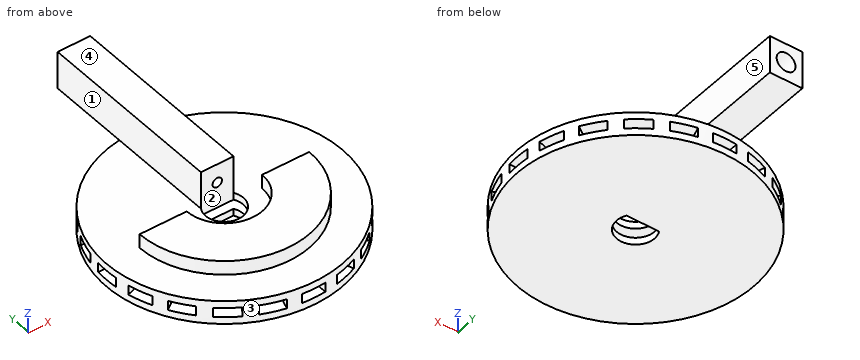
Autodesk Inventor part; units mm, degrees
ref_plane "Work Plane1" through (0, 25, 0) normal (0, 1, 0) x (-1, 0, 0)
ref_plane "YZ Plane" through (0, 0, 0) normal (1, 0, 0) x (0, 1, 0)
ref_plane "XY Plane" through (0, 0, 0) normal (0, 0, 1) x (1, 0, 0)
sketch "Sketch1" plane through (0, 0, 0) normal (0, 0, 1) x (1, 0, 0)
  circle A0 centre (0, 0) radius 25
  circle A1 centre (0, 0) radius 4
  line L0 (-3.4641, 2) -> (3.4641, 2)
  dimension "d0" = 50
  dimension "d1" = 8
  dimension "d2" = 2
extrude "Extrusion1" add sketch "Sketch1" along normal blind 5 contours A0 | L0 A1 picked at (-0.1548, 2.6577)
ref_plane "Work Plane1" through (0, 25, 0) normal (0, 1, 0) x (-1, 0, 0)
sketch "Sketch3" plane through (0, 25, 0) normal (0, 1, 0) x (-1, 0, 0)
  line L0 (2.5, 1.5) -> (-2.5, 1.5)
  line L1 (-2.5, 1.5) -> (-2.5, 3.5)
  line L2 (-2.5, 3.5) -> (2.5, 3.5)
  line L3 (2.5, 3.5) -> (2.5, 1.5)
  line L4 (25, 0) -> (25, 5) construction
  point P0 (0, 0)
  point P1 (0, 1.5)
  point P2 (2.5, 2.5)
  point P3 (25, 2.5)
  dimension "d12" = 5
  dimension "d13" = 2
extrude "Extrusion2" cut sketch "Sketch3" against normal blind 25
pattern_circular "Circular Pattern1" count 20 over 360 about axis through (0, 0, -10) along (0, 0, 1) of "Extrusion2"
sketch "Sketch4" plane through (0, 0, 5) normal (0, 0, 1) x (1, 0, 0)
  line L0 (-3.4641, 2) -> (3.4641, 2)
  line L1 (-3.4641, 2) -> (3.4641, 2)
  line L2 (3.4641, 2) -> (3.4641, 42)
  line L3 (3.4641, 42) -> (-3.4641, 42)
  line L4 (-3.4641, 42) -> (-3.4641, 2)
  point P0 (0, 0)
  dimension "d19" = 40
  dimension "d20" = 6.9282
extrude "Extrusion3" add sketch "Sketch4" along normal blind 8
sketch "Sketch5" plane through (-3.4641, 42, 5) normal (0, 1, 0) x (1, 0, 0)
  circle A0 centre (3.4641, -4) radius 2
  line L0 (6.9282, 0) -> (0, 0) construction
  line L1 (0, 0) -> (0, -8) construction
  line L2 (6.9282, -8) -> (0, -8) construction
  line L3 (6.9282, 0) -> (6.9282, -8) construction
  point P0 (3.4641, 5)
  point P1 (6.9282, -4)
  point P2 (3.4641, -8)
  dimension "d23" = 4
sketch "Sketch6" plane through (-3.4641, 2, 3.5) normal (0, -1, 0) x (1, 0, 0)
  circle A0 centre (3.4641, 5.5) radius 1
  line L0 (0, 9.5) -> (6.9282, 9.5)
  line L1 (6.9282, 1.5) -> (6.9282, 9.5)
  point P0 (3.4641, -3.5)
  point P1 (3.4641, 9.5)
  point P2 (6.9282, 5.5)
  dimension "d24" = 2
loft "Loft1" cut profiles "Sketch5", "Sketch6"
sketch "Sketch7" plane through (0, 0, 0) normal (0, 1, 0) x (-1, 0, 0)
  line L0 (25, 5) -> (-25, 5) construction
  line L1 (8, 5) -> (18, 5)
  line L2 (18, 5) -> (18, 8)
  line L3 (18, 8) -> (8, 8)
  line L4 (8, 8) -> (8, 5)
  line L5 (-10.0643, 3.5) -> (-5.3091, 3.5) construction
  line L6 (-5.3091, 3.5) -> (-5.3091, 1.5) construction
  line L7 (-5.3091, 1.5) -> (-10.0643, 1.5) construction
  line L8 (-10.0643, 1.5) -> (-10.0643, 3.5) construction
  line L9 (-24.8747, 1.5) -> (-24.8747, 1.5) construction
  line L10 (-24.8747, 1.5) -> (-24.8747, 3.5) construction
  line L11 (-24.8747, 3.5) -> (-24.8747, 3.5) construction
  line L12 (-24.8747, 3.5) -> (-24.8747, 1.5) construction
  line L13 (-24.4298, 1.5) -> (-22.8847, 1.5) construction
  line L14 (-22.8847, 1.5) -> (-22.8847, 3.5) construction
  line L15 (-22.8847, 3.5) -> (-24.4298, 3.5) construction
  line L16 (-24.4298, 3.5) -> (-24.4298, 1.5) construction
  line L17 (-21.5935, 1.5) -> (-18.6546, 1.5) construction
  line L18 (-18.6546, 1.5) -> (-18.6546, 3.5) construction
  line L19 (-18.6546, 3.5) -> (-21.5935, 3.5) construction
  line L20 (-21.5935, 3.5) -> (-21.5935, 1.5) construction
  line L21 (-16.6435, 1.5) -> (-12.5984, 1.5) construction
  line L22 (-12.5984, 1.5) -> (-12.5984, 3.5) construction
  line L23 (-12.5984, 3.5) -> (-16.6435, 3.5) construction
  line L24 (-16.6435, 3.5) -> (-16.6435, 1.5) construction
  line L25 (-10.0643, 1.5) -> (-5.3091, 1.5) construction
  line L26 (-5.3091, 1.5) -> (-5.3091, 3.5) construction
  line L27 (-5.3091, 3.5) -> (-10.0643, 3.5) construction
  line L28 (-10.0643, 3.5) -> (-10.0643, 1.5) construction
  line L29 (10.0643, 1.5) -> (5.3091, 1.5) construction
  line L30 (5.3091, 1.5) -> (5.3091, 3.5) construction
  line L31 (5.3091, 3.5) -> (10.0643, 3.5) construction
  line L32 (10.0643, 3.5) -> (10.0643, 1.5) construction
  line L33 (-12.5984, 1.5) -> (-16.6435, 1.5) construction
  line L34 (-16.6435, 1.5) -> (-16.6435, 3.5) construction
  line L35 (-16.6435, 3.5) -> (-12.5984, 3.5) construction
  line L36 (-12.5984, 3.5) -> (-12.5984, 1.5) construction
  line L37 (-18.6546, 1.5) -> (-21.5935, 1.5) construction
  line L38 (-21.5935, 1.5) -> (-21.5935, 3.5) construction
  line L39 (-21.5935, 3.5) -> (-18.6546, 3.5) construction
  line L40 (-18.6546, 3.5) -> (-18.6546, 1.5) construction
  line L41 (-22.8847, 1.5) -> (-24.4298, 1.5) construction
  line L42 (-24.4298, 1.5) -> (-24.4298, 3.5) construction
  line L43 (-24.4298, 3.5) -> (-22.8847, 3.5) construction
  line L44 (-22.8847, 3.5) -> (-22.8847, 1.5) construction
  line L45 (12.5984, 3.5) -> (16.6435, 3.5) construction
  line L46 (16.6435, 3.5) -> (16.6435, 1.5) construction
  line L47 (16.6435, 1.5) -> (12.5984, 1.5) construction
  line L48 (12.5984, 1.5) -> (12.5984, 3.5) construction
  line L49 (18.6546, 3.5) -> (21.5935, 3.5) construction
  line L50 (21.5935, 3.5) -> (21.5935, 1.5) construction
  line L51 (21.5935, 1.5) -> (18.6546, 1.5) construction
  line L52 (18.6546, 1.5) -> (18.6546, 3.5) construction
  line L53 (22.8847, 3.5) -> (24.4298, 3.5) construction
  line L54 (24.4298, 3.5) -> (24.4298, 1.5) construction
  line L55 (24.4298, 1.5) -> (22.8847, 1.5) construction
  line L56 (22.8847, 1.5) -> (22.8847, 3.5) construction
  line L57 (24.8747, 3.5) -> (24.8747, 3.5) construction
  line L58 (24.8747, 3.5) -> (24.8747, 1.5) construction
  line L59 (24.8747, 1.5) -> (24.8747, 1.5) construction
  line L60 (24.8747, 1.5) -> (24.8747, 3.5) construction
  line L61 (24.4298, 3.5) -> (22.8847, 3.5) construction
  line L62 (22.8847, 3.5) -> (22.8847, 1.5) construction
  line L63 (22.8847, 1.5) -> (24.4298, 1.5) construction
  line L64 (24.4298, 1.5) -> (24.4298, 3.5) construction
  line L65 (21.5935, 3.5) -> (18.6546, 3.5) construction
  line L66 (18.6546, 3.5) -> (18.6546, 1.5) construction
  line L67 (18.6546, 1.5) -> (21.5935, 1.5) construction
  line L68 (21.5935, 1.5) -> (21.5935, 3.5) construction
  line L69 (16.6435, 3.5) -> (12.5984, 3.5) construction
  line L70 (12.5984, 3.5) -> (12.5984, 1.5) construction
  line L71 (12.5984, 1.5) -> (16.6435, 1.5) construction
  line L72 (16.6435, 1.5) -> (16.6435, 3.5) construction
  line L73 (10.0643, 3.5) -> (5.3091, 3.5) construction
  line L74 (5.3091, 3.5) -> (5.3091, 1.5) construction
  line L75 (5.3091, 1.5) -> (10.0643, 1.5) construction
  line L76 (10.0643, 1.5) -> (10.0643, 3.5) construction
  line L77 (2.5, 3.5) -> (-2.5, 3.5) construction
  line L78 (-2.5, 3.5) -> (-2.5, 1.5) construction
  line L79 (-2.5, 1.5) -> (2.5, 1.5) construction
  line L80 (2.5, 1.5) -> (2.5, 3.5) construction
  line L81 (-2.5, 3.5) -> (2.5, 3.5) construction
  line L82 (2.5, 3.5) -> (2.5, 1.5) construction
  line L83 (2.5, 1.5) -> (-2.5, 1.5) construction
  line L84 (-2.5, 1.5) -> (-2.5, 3.5) construction
  line L85 (3.4641, 5) -> (-3.4641, 5) construction
  line L86 (-3.4641, 5) -> (3.4641, 5) construction
  line L87 (-25, 0) -> (25, 0) construction
  circle A0 centre (0, 9) radius 1 construction
  line L88 (3.4641, 3.5) -> (-3.4641, 3.5) construction
  line L89 (-3.4641, 3.5) -> (-3.4641, 5) construction
  line L90 (-3.4641, 5) -> (-3.4641, 13) construction
  line L91 (3.4641, 13) -> (-3.4641, 13) construction
  line L92 (3.4641, 5) -> (3.4641, 13) construction
  line L93 (3.4641, 3.5) -> (3.4641, 5) construction
  line L94 (0, -2.6) -> (0, 15.6)
  point P0 (0, 0)
  dimension "d29" = 8
  dimension "d30" = 3
  dimension "d31" = 10
revolve "Revolution1" add sketch "Sketch7" angle 180 about axis through (0, 0, -10) along (0, 0, 1)
properties part number "Parcial3_Repo"
Work out the finished part from the listing and answer in its coordinate system (mm). Face numbers are marked on the shaded views. A direction names the side the tool comes from. Round coordinates to 2 decimals unless told otherwise and drop trailing zeros. Order: outer loops, then holes, each group sorted by start corner. A loop starts at its lowest first (then second) coordinate and runs counter-clockwise, first axis right, second up. Notation, with made-up numbers: M -23,27.5 L 26,27.5 A9 cw 26,40.5 Z; hole C 5.25,16 d4. An arc over 180 degrees is marked long. One line per item, written item: value.
Q1. Find section C-C on y = 28. Write down the section's boundary in (x, z).
Derived:
outline: M -3.46,5 L 3.46,5 L 3.46,13 L -3.46,13 Z; hole C 0,9 d3.3
Q2. Determine the mould class of the marked faces 1, 2 and 3 for opening direction Y: released by +Y, released by -Y, zero draft, split by the parting line, or undercut.
Derived:
face 1: zero draft
face 2: undercut
face 3: split by the parting line
Q3. Find section D-D on x = 20. Write down the section's boundary in (y, z).
Derived:
outline: M -15,0 L 15,0 L 15,1.5 L 11.44,1.5 L 11.44,3.5 L 15,3.5 L 15,5 L -15,5 L -15,3.5 L -11.44,3.5 L -11.44,1.5 L -15,1.5 Z; hole M -9.13,1.5 L -3.87,1.5 L -3.87,3.5 L -9.13,3.5 Z; hole M -2.5,1.5 L 2.5,1.5 L 2.5,3.5 L -2.5,3.5 Z; hole M 3.87,1.5 L 9.13,1.5 L 9.13,3.5 L 3.87,3.5 Z
Q4. Find section A-A on x = 0. Write down the section's boundary in (y, z), then the cut area to 3 significant figures.
Derived:
outline: M -25,0 L -4,0 L -4,1.5 L -25,1.5 Z; M -25,3.5 L -4,3.5 L -4,5 L -8,5 L -8,8 L -18,8 L -18,5 L -25,5 Z; M 2,0 L 25,0 L 25,1.5 L 2,1.5 Z; M 2,3.5 L 25,3.5 L 25,5 L 42,5 L 42,7 L 2,8 Z; M 2,10 L 42,11 L 42,13 L 2,13 Z
area: 362 mm²
Q5. Find section B-B on y = -1. Write down the section's boundary in (x, z), then the cut area to 3 significant figures.
Derived:
outline: M -24.98,0 L -3.87,0 L -3.87,1.5 L -24.98,1.5 Z; M -24.98,3.5 L -3.87,3.5 L -3.87,5 L -7.94,5 L -7.94,8 L -17.97,8 L -17.97,5 L -24.98,5 Z; M 3.87,0 L 24.98,0 L 24.98,1.5 L 3.87,1.5 Z; M 3.87,3.5 L 24.98,3.5 L 24.98,5 L 17.97,5 L 17.97,8 L 7.94,8 L 7.94,5 L 3.87,5 Z
area: 187 mm²
Q6. Straight lines are drawn through the part: line 1 (X direction, y = 0, z = 4.2); line 2 (Y direction, x = 0, z = 0.65); line 3 (Z direction, x = 16.5, y = -14). For each, find the intervals that lie inside material, in ascending order.
Derived:
line 1: -25 to -4, 4 to 25
line 2: -25 to -4, 2 to 25
line 3: 0 to 1.5, 3.5 to 5
Q7. Flat-ended cylindrical pins translate along their axes: pin 1 (4 mm diameter, centred on y = 22, z = 10.5, fed in from +X); pin 2 (5.5 mm diameter, centred on x = -8, y = -6, fed in from +Z); pin 3 (5 mm diameter, centred on y = 11, z = 5, fed in from -X). Find the tip coordinate at first contact, or state that the pin passes through.
Derived:
pin 1: x = 3.46
pin 2: z = 8
pin 3: x = -23.51
Q8. For the marked faces 4 and 5, determine the directions among +Z, -Z, +X, -X, +Y, -Y from which every point of the face is accessible in a straight line to the end or side of a thin tool.
Derived:
face 4: +Z, +X, -X, +Y, -Y
face 5: +Z, +X, +Y
